Check sheet for the modelled part. Datum: model origin and axes. Units: mm. Face numbers are marked on the shaded views. A direction names the side the tool comes from. Coordinates: 2 decimals unless noted, no trailing zeros. Loops run counter-clockwise (first coordinate to the right, second up) from the corner with the lowest first, then second, coordinate; pieces in that order, holes last. Notation, with made-up numbers: (-27.5, 51.25) -> (21.5, 51.25) arc R35 cw to (21.5, 83.25) -> close; hole circle Ø6 at (-29, 4.5). An arc over 180 degrees is marked (long way). Use CSV: the item, a comma, the result in double quotes.
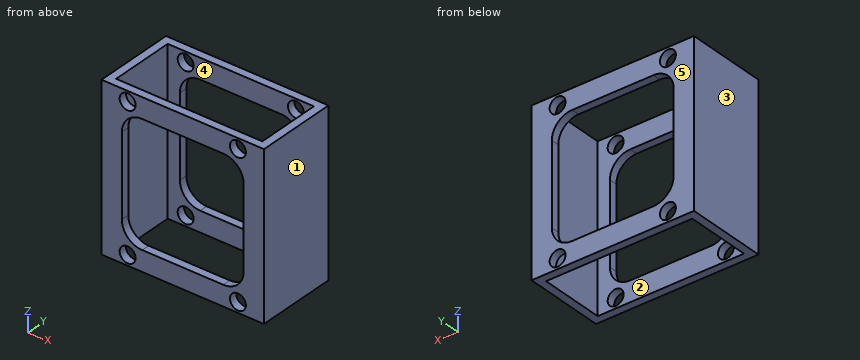
```python
from build123d import *

# Parameters (mm, degrees)
SKETCH1_W           = 50.8
SKETCH1_H           = 25.4
SKETCH1_W_2         = 45.72
SKETCH1_H_2         = 20.32
EXTRUDE_THIN1_DEPTH = 50.8
CUT_EXTRUDE1_DEPTH  = 26.4
SKETCH3_R           = 2.4892
CUT_EXTRUDE2_DEPTH  = 26.4


with BuildPart() as part:
    # Sketch1 → Extrude-Thin1 (new body)
    with BuildSketch(Plane.XY):
        Rectangle(SKETCH1_W, SKETCH1_H)
        Rectangle(SKETCH1_W_2, SKETCH1_H_2, mode=Mode.SUBTRACT)
    extrude(amount=EXTRUDE_THIN1_DEPTH)

    # Sketch2 → Cut-Extrude1 (cut, through all)
    with BuildSketch(Plane(origin=(0, 12.7, 0), x_dir=(1, 0, 0), z_dir=(0, 1, 0))):
        with BuildLine():
            ThreePointArc((12.7, -44.45), (17.190128061, -42.590128061), (19.05, -38.1))
            Line((19.05, -38.1), (19.05, -12.7))
            ThreePointArc((19.05, -12.7), (17.190128061, -8.209871939), (12.7, -6.35))
            Line((12.7, -6.35), (-12.7, -6.35))
            ThreePointArc((-12.7, -6.35), (-17.190128061, -8.209871939), (-19.05, -12.7))
            Line((-19.05, -12.7), (-19.05, -38.1))
            ThreePointArc((-19.05, -38.1), (-17.190128061, -42.590128061), (-12.7, -44.45))
            Line((-12.7, -44.45), (12.7, -44.45))
        make_face()
    extrude(amount=-CUT_EXTRUDE1_DEPTH, mode=Mode.SUBTRACT)

    # Sketch3 → Cut-Extrude2 (cut, through all)
    with BuildSketch(Plane(origin=(0, 12.7, 0), x_dir=(1, 0, 0), z_dir=(0, 1, 0))):
        with Locations((-17.2466, -47.625)):
            Circle(SKETCH3_R)
        with Locations((17.2466, -47.625)):
            Circle(SKETCH3_R)
        with Locations((17.2466, -3.175)):
            Circle(SKETCH3_R)
        with Locations((-17.2466, -3.175)):
            Circle(SKETCH3_R)
    extrude(amount=-CUT_EXTRUDE2_DEPTH, mode=Mode.SUBTRACT)


solid = part.part
```
1) Cross-section at A-A on y = 0.5. Record the boundary of the cut face in (x, z).
Answer below:
outline,"(-25.4, 0) -> (-22.86, 0) -> (-22.86, 50.8) -> (-25.4, 50.8) -> close; (22.86, 0) -> (25.4, 0) -> (25.4, 50.8) -> (22.86, 50.8) -> close"
2) Cross-section at D-D on z = 47. Record the boundary of the cut face in (x, y), and give its area (3 significant figures).
Answer below:
outline,"(-25.4, -12.7) -> (-19.66, -12.7) -> (-19.66, -10.16) -> (-22.86, -10.16) -> (-22.86, 10.16) -> (-19.66, 10.16) -> (-19.66, 12.7) -> (-25.4, 12.7) -> close; (-14.84, -12.7) -> (14.84, -12.7) -> (14.84, -10.16) -> (-14.84, -10.16) -> close; (-14.84, 10.16) -> (14.84, 10.16) -> (14.84, 12.7) -> (-14.84, 12.7) -> close; (19.66, -12.7) -> (25.4, -12.7) -> (25.4, 12.7) -> (19.66, 12.7) -> (19.66, 10.16) -> (22.86, 10.16) -> (22.86, -10.16) -> (19.66, -10.16) -> close"
area,"312 mm²"
3) Cross-section at B-B on z = 32.5. Record the boundary of the cut face in (x, y), and give its area (3 significant figures).
Answer below:
outline,"(-25.4, -12.7) -> (-19.05, -12.7) -> (-19.05, -10.16) -> (-22.86, -10.16) -> (-22.86, 10.16) -> (-19.05, 10.16) -> (-19.05, 12.7) -> (-25.4, 12.7) -> close; (19.05, -12.7) -> (25.4, -12.7) -> (25.4, 12.7) -> (19.05, 12.7) -> (19.05, 10.16) -> (22.86, 10.16) -> (22.86, -10.16) -> (19.05, -10.16) -> close"
area,"168 mm²"
4) Go/stop test with flat-tipped pins: pin 1 Ø8 at (x, z) = (-17.25, 47.62) entering from -Y; pin 2 Ø3 at (x, z) = (17.25, 47.62) entering from -Y. Record where each tip stops, or that it passes through.
Answer below:
pin 1,"stops at y = -12.7"
pin 2,"passes through"
5) Access from +Z, -Z, +X, -X, +Y, -Y to the whole of each face (thin tool, end or side, straight path). Record for the marked faces 1 and 2.
Answer below:
face 1,"+Z, -Z, +X, +Y, -Y"
face 2,"+Z, -Z"
6) Cross-section at C-C on x = -8. Record the boundary of the cut face in (y, z), and give its area (3 significant figures).
Answer below:
outline,"(-12.7, 0) -> (-10.16, 0) -> (-10.16, 6.35) -> (-12.7, 6.35) -> close; (-12.7, 44.45) -> (-10.16, 44.45) -> (-10.16, 50.8) -> (-12.7, 50.8) -> close; (10.16, 0) -> (12.7, 0) -> (12.7, 6.35) -> (10.16, 6.35) -> close; (10.16, 44.45) -> (12.7, 44.45) -> (12.7, 50.8) -> (10.16, 50.8) -> close"
area,"64.5 mm²"
7) Draft check along Y on the marked faces 3, 4 and 5. Enter one of: released by +Y, released by -Y, zero draft, split by the parting line, or undercut.
Answer below:
face 3,"zero draft"
face 4,"undercut"
face 5,"released by +Y"
8) Thickness scan on line 1 along X through (y, z) = (-11.25, 14); line 2 along X through (y, z) = (2.25, 8.5); line 3 along Y through (x, z) = (13, 47). Record the ranges inside material, lowest first. Write a range as from..to.
Answer below:
line 1,"x = -25.4..-19.05, 19.05..25.4"
line 2,"x = -25.4..-22.86, 22.86..25.4"
line 3,"y = -12.7..-10.16, 10.16..12.7"
